Here's how the part is built. I have some questions about the finished solid (model axes, mm). Coordinates: 2 decimals unless noted, no trailing zeros. Order: outer loops, then holes, each group sorted by start corner. A loop starts at its lowest first (then second) coordinate and runs counter-clockwise, first axis right, second up. Notation, with made-up numbers: (73, -14) - (88, -14) arc R35 cw to (88, 24) - close; hole circle Ø1 at (66.5, -37). An arc over 180 degrees is marked (long way). Answer in a Markdown table with one row per item. Add a question column.
Item 1: Will these pins go through, and if not, where does the flat tip stop? pin 1 Ø0.9 at (x, z) = (62.5, 2) entering from -Y; pin 2 Ø0.9 at (y, z) = (18, 2) entering from -X; pin 3 Ø0.9 at (x, z) = (62.5, 1.5) entering from +Y.
Item 2: I want a section at B-B (x = -35.25). Please give me the cut outline in (y, z).
Item 3: I want a section at A-A (y = -18.9). Please give me the cut outline in (x, z), plus the area to 3 significant figures.
Item 4: I want a section at C-C (x = -20). Please give me the cut outline in (y, z), plus the area to 3 significant figures.
Item 5: I want a section at D-D (z = 1.6). Please give me the cut outline in (x, y).
Item 6: If I drill on line 1 along Y through (x, z) = (35.25, 2.3); line 2 along X through (y, z) = (5, 0.15); line 3 along X through (y, z) = (-1, 1.9), over which ranges is the centre line in solid material (lowest first)? Write a range as from..to.
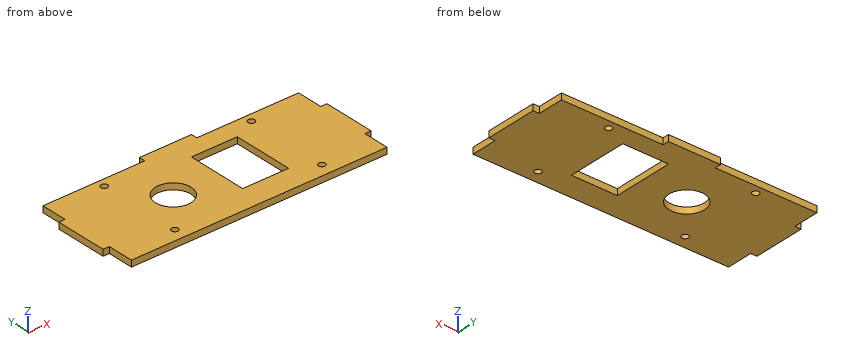
```python
from build123d import *

# Parameters (mm, degrees)
BOSS_EXTRU_1_DEPTH = 3
SKETCH1_R          = 1.6
CUT_EXTRUDE1_DEPTH = 71.150285103
SKETCH2_R          = 1.6
CUT_EXTRUDE2_DEPTH = 71.150285103
SKETCH3_R          = 1.6
CUT_EXTRUDE3_DEPTH = 71.150285103
SKETCH4_W          = 22
SKETCH4_H          = 29
CUT_EXTRUDE4_DEPTH = 71.150285103
SKETCH5_R          = 8.5
CUT_EXTRUDE5_DEPTH = 71.150285103


with BuildPart() as part:
    # Esquisse1 → Boss.-Extru.1 (new body)
    with BuildSketch(Plane.XY):
        Polygon((61.25, -25), (-61.25, -25), (-61.25, -12.5), (-64.25, -12.5), (-64.25, 12.5), (-61.25, 12.5), (-61.25, 25), (-29.85, 25), (-26.65, 25), (-12.5, 25), (-12.5, 28), (12.5, 28), (12.5, 25), (26.65, 25), (29.85, 25), (61.25, 25), (61.25, 12.5), (64.25, 12.5), (64.25, -12.5), (61.25, -12.5), align=None)
    extrude(amount=BOSS_EXTRU_1_DEPTH)

    # Sketch1 → Cut-Extrude1 (cut, through all)
    with BuildSketch(Plane(origin=(0, 0, 0), x_dir=(-1, 0, 0), z_dir=(0, 0, -1))):
        with Locations((35.25, 21)):
            Circle(SKETCH1_R)
    extrude(amount=-CUT_EXTRUDE1_DEPTH, mode=Mode.SUBTRACT)

    # Sketch2 → Cut-Extrude2 (cut, through all)
    with BuildSketch(Plane(origin=(0, 0, 0), x_dir=(-1, 0, 0), z_dir=(0, 0, -1))):
        with Locations((-35.25, 21)):
            Circle(SKETCH2_R)
    extrude(amount=-CUT_EXTRUDE2_DEPTH, mode=Mode.SUBTRACT)

    # Sketch3 → Cut-Extrude3 (cut, through all)
    with BuildSketch(Plane(origin=(0, 0, 0), x_dir=(-1, 0, 0), z_dir=(0, 0, -1))):
        with Locations((35.25, -18.9)):
            Circle(SKETCH3_R)
        with Locations((-35.25, -18.9)):
            Circle(SKETCH3_R)
    extrude(amount=-CUT_EXTRUDE3_DEPTH, mode=Mode.SUBTRACT)

    # Sketch4 → Cut-Extrude4 (cut, through all)
    with BuildSketch(Plane.XY.offset(3)):
        with Locations((13.25, 1.5)):
            Rectangle(SKETCH4_W, SKETCH4_H)
    extrude(amount=-CUT_EXTRUDE4_DEPTH, mode=Mode.SUBTRACT)

    # Sketch5 → Cut-Extrude5 (cut, through all)
    with BuildSketch(Plane.XY.offset(3)):
        with Locations((-20, 0)):
            Circle(SKETCH5_R)
    extrude(amount=-CUT_EXTRUDE5_DEPTH, mode=Mode.SUBTRACT)


solid = part.part
```
Values follow:
| question | item | result |
|---|---|---|
| 1 | pin 1 | stops at y = -12.5 |
| 1 | pin 2 | stops at x = -61.25 |
| 1 | pin 3 | stops at y = 12.5 |
| 2 | outline | (-25, 0) - (-20.5, 0) - (-20.5, 3) - (-25, 3) - close; (-17.3, 0) - (19.4, 0) - (19.4, 3) - (-17.3, 3) - close; (22.6, 0) - (25, 0) - (25, 3) - (22.6, 3) - close |
| 3 | outline | (-61.25, 0) - (-36.85, 0) - (-36.85, 3) - (-61.25, 3) - close; (-33.65, 0) - (33.65, 0) - (33.65, 3) - (-33.65, 3) - close; (36.85, 0) - (61.25, 0) - (61.25, 3) - (36.85, 3) - close |
| 3 | area | 348 mm^2 |
| 4 | outline | (-25, 0) - (-8.5, 0) - (-8.5, 3) - (-25, 3) - close; (8.5, 0) - (25, 0) - (25, 3) - (8.5, 3) - close |
| 4 | area | 99.0 mm^2 |
| 5 | outline | (-64.25, -12.5) - (-61.25, -12.5) - (-61.25, -25) - (61.25, -25) - (61.25, -12.5) - (64.25, -12.5) - (64.25, 12.5) - (61.25, 12.5) - (61.25, 25) - (12.5, 25) - (12.5, 28) - (-12.5, 28) - (-12.5, 25) - (-61.25, 25) - (-61.25, 12.5) - (-64.25, 12.5) - close; hole circle Ø3.2 at (-35.25, -18.9); hole circle Ø3.2 at (-35.25, 21); hole circle Ø17 at (-20, 0); hole (2.25, -13) - (24.25, -13) - (24.25, 16) - (2.25, 16) - close; hole circle Ø3.2 at (35.25, -18.9); hole circle Ø3.2 at (35.25, 21) |
| 6 | line 1 | y = -25..-20.5, -17.3..19.4, 22.6..25 |
| 6 | line 2 | x = -64.25..-26.87, -13.13..2.25, 24.25..64.25 |
| 6 | line 3 | x = -64.25..-28.44, -11.56..2.25, 24.25..64.25 |
